Can you work these out from the drawing? Everything is in mm from the part's minimum corner. Round coordinates to 2 decimals unless told otherwise and drop trailing zeros. Order: outer loops, then holes, each group sorted by start corner. A loop starts at its lowest first (then second) coordinate and runs counter-clockwise, first axis right, second up. Notation, with made-up numbers: (51, -34) -> (85, -34) arc R32 cw to (85, -3) -> close; hole circle Ø10 at (-18, -30.75). An arc over 180 degrees is marked (long way). One line per item, written item: value.
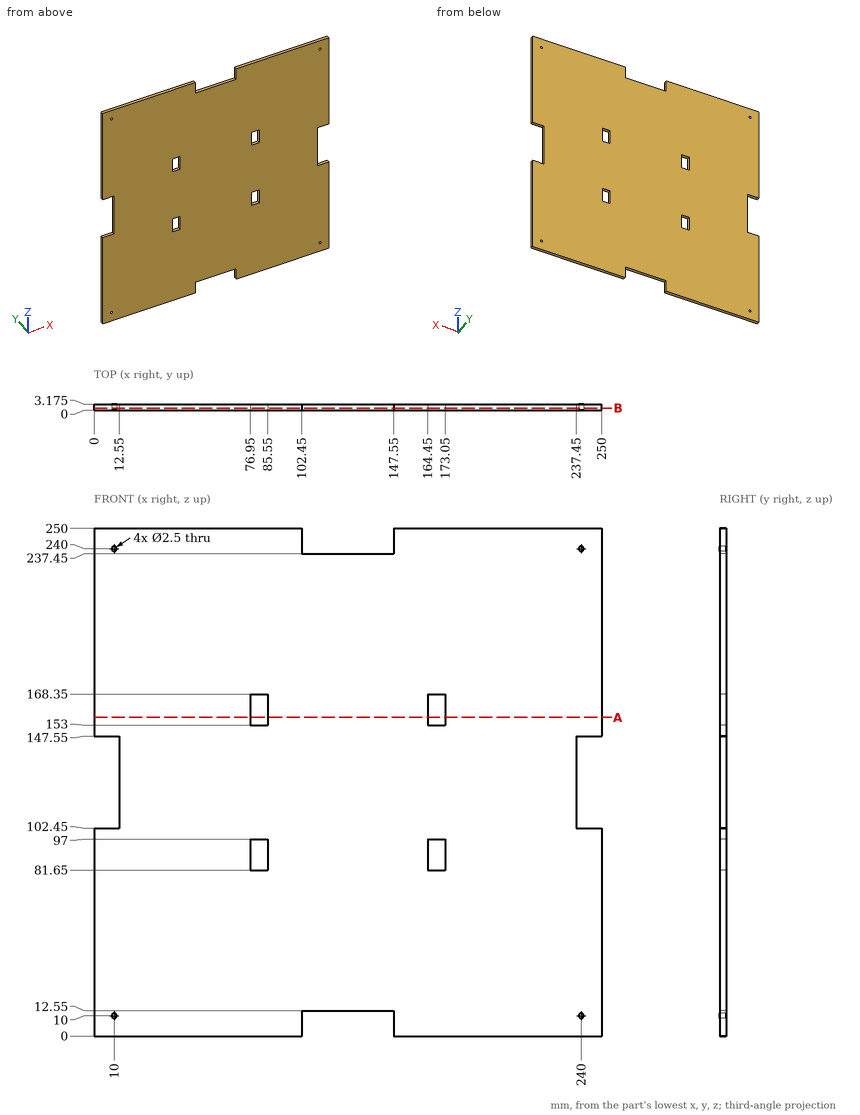
Q1. I want a section at B-B on y = 1.1. Give the number of separate pieces and of enclosed holes in the cut face, plus the area to 3 significant figures.
Answers below:
separate pieces: 1
enclosed holes: 8
area: 59,700 mm^2
Q2. Please list where these lines run through material, in increasing order: line 1 along X through (y, z) = (1.9, 240); line 2 along X through (y, z) = (2.55, 114).
Answers below:
line 1: 0 to 8.75, 11.25 to 102.45, 147.55 to 238.75, 241.25 to 250
line 2: 12.55 to 237.45
Q3. Will these pins go through, and if not, where does the flat tip stop? pin 1 Ø1.5 at (x, z) = (240, 240) entering from -Y; pin 2 Ø1.6 at (y, z) = (1.5, 129) entering from -X.
Answers below:
pin 1: through
pin 2: x = 12.55
Q4. I want a section at A-A on z = 157. List the corners of the cut face in (x, y) for me (3 decimals), plus the area to 3 significant figures.
Answers below:
outline: (0, 0) -> (76.95, 0) -> (76.95, 3.175) -> (0, 3.175) -> close; (85.55, 0) -> (164.45, 0) -> (164.45, 3.175) -> (85.55, 3.175) -> close; (173.05, 0) -> (250, 0) -> (250, 3.175) -> (173.05, 3.175) -> close
area: 739 mm^2
